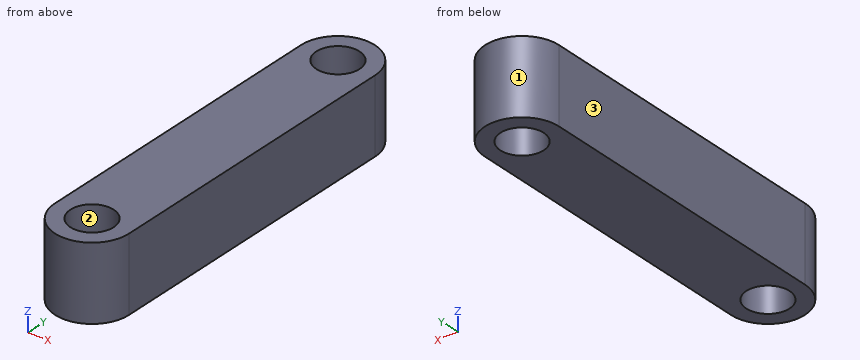
```python
from build123d import *

# Parameters (mm, degrees)
SKETCH1_R           = 3.5
BOSS_EXTRUDE1_DEPTH = 12


with BuildPart() as part:
    # Sketch1 → Boss-Extrude1 (new body)
    with BuildSketch(Plane.XY):
        with BuildLine():
            Line((-6, 0), (-6, -50))
            ThreePointArc((-6, -50), (0, -56), (6, -50))
            Line((6, -50), (6, 0))
            ThreePointArc((6, 0), (0, 6), (-6, 0))
        make_face()
        Circle(SKETCH1_R, mode=Mode.SUBTRACT)
        with Locations((0, -50)):
            Circle(SKETCH1_R, mode=Mode.SUBTRACT)
    extrude(amount=-BOSS_EXTRUDE1_DEPTH)


solid = part.part
```
Work out the finished part from the listing and answer in its coordinate system (mm). Face numbers are marked on the shaded views. Round coordinates to 2 decimals unless told otherwise and drop trailing zeros. Loops run counter-clockwise (first coordinate to the right, second up) from the corner with the lowest first, then second, coordinate; pieces in that order, holes last. Notation, with made-up numbers: M 40,-0.75 L 98,-0.75 A13 cw 98,17.25 Z; hole C 18,50.25 d9. An arc over 180 degrees is marked long. Use CSV: the item, a comma, the result in double quotes.
Q1. Section C-C, the plane y = -51 is taken. Determine the outline of the cut face in (x, z), then the cut area to 3 significant figures.
Determined:
outline,"M -5.92,-12 L -3.35,-12 L -3.35,0 L -5.92,0 Z; M 3.35,-12 L 5.92,-12 L 5.92,0 L 3.35,0 Z"
area,"61.5 mm2"
Q2. Section B-B, the plane z = -7 is taken. Determine the outline of the cut face in (x, y).
Determined:
outline,"M -6,-50 A6 ccw 6,-50 L 6,0 A6 ccw -6,0 Z; hole C 0,-50 d7; hole C 0,0 d7"
Q3. The mould has two halves that part along Y. Classify the marked faces 1, 2 and 3: pulls with the +Y half, pulls with the -Y half, needs draft (parallel to the pull), parting line crosses it, or undercut.
Determined:
face 1,"pulls with the +Y half"
face 2,"undercut"
face 3,"needs draft"
Q4. Section A-A, the plane x = 0 is taken. Determine the outline of the cut face in (y, z), then the cut area to 3 significant figures.
Determined:
outline,"M -56,-12 L -53.5,-12 L -53.5,0 L -56,0 Z; M -46.5,-12 L -3.5,-12 L -3.5,0 L -46.5,0 Z; M 3.5,-12 L 6,-12 L 6,0 L 3.5,0 Z"
area,"576 mm2"
Q5. Section D-D, the plane x = 2.25 is taken. Determine the outline of the cut face in (y, z).
Determined:
outline,"M -55.56,-12 L -52.68,-12 L -52.68,0 L -55.56,0 Z; M -47.32,-12 L -2.68,-12 L -2.68,0 L -47.32,0 Z; M 2.68,-12 L 5.56,-12 L 5.56,0 L 2.68,0 Z"
Q6. Consider L1, parallel to Y at x = 0, z = -6.25; L2, parallel to Y at x = 0.75, z = -4.5; L3, parallel to X at y = -48.5, z = -4.75. Determine where each line is inside the solid, lowest interval first.
Determined:
L1,"-56 to -53.5, -46.5 to -3.5, 3.5 to 6"
L2,"-55.95 to -53.42, -46.58 to -3.42, 3.42 to 5.95"
L3,"-6 to -3.16, 3.16 to 6"
Q7. Each of these flat-tipped pins is pushed along its axis until it touches: pin 1 (2 mm diameter, centred on x = 2.5, z = -5.5, fed in from +Y); pin 2 (1.5 mm diameter, centred on x = -2.5, z = -6, fed in from +Y). Where does it stop, or does it pass through?
Determined:
pin 1,"y = 5.81"
pin 2,"y = 5.74"
